Work out the finished part from the listing and answer in its coordinate system (mm). A direction names the side the tool comes from. Give positions to 0.01 mm unless a question says otherwise; leave off trailing zeros. Order: outer loops, then holes, each group sorted by start corner. A loop starts at its lowest first (then second) coordinate and runs counter-clockwise, first axis right, second up. Notation, with made-up numbers: (-30, 35.25) - (10, 35.25) arc R11 cw to (10, 49.25) - close; hole circle Ø8 at (77, -37.75). An arc over 180 degrees is marked (long way). Put each result on its own line as item: value.
```python
from build123d import *

# Parameters (mm, degrees)
SKETCH_1_R             = 1.6
SM_BASE_FLANGE_1_DEPTH = 0.9
OTHER_START            = -10
OTHER_1_DEPTH          = 20
OTHER_1_2_DEPTH        = 20


# Read off the part's stored shape, not the designer's step: 褶边1
# Sheet-metal steps are written as plain solids
with BuildPart() as part:
    # Sketch 1 → 基体-法兰1 (new body)
    with BuildSketch(Plane.XY):
        with BuildLine():
            Line((10, 0), (-10, 0))
            Line((-10, 0), (-10, 10))
            ThreePointArc((-10, 10), (0, 14.142135624), (10, 10))
            Line((10, 10), (10, 0))
        make_face()
        with Locations((-6.5, 6.5)):
            Circle(SKETCH_1_R, mode=Mode.SUBTRACT)
        with Locations(Location((6.5, 6.5, 0), (0, 0, 180))):
            Circle(SKETCH_1_R, mode=Mode.SUBTRACT)
    extrude(amount=-SM_BASE_FLANGE_1_DEPTH)

    # Other 1 outline → Other 1 (cut)
    with BuildSketch(Plane.YZ.offset(OTHER_START)):
        with BuildLine():
            ThreePointArc((2.4, -0.9), (1.360769515, -0.663330765), (0.5265006, 0))
            Line((0.5265006, 0), (0, 0))
            Line((0, 0), (0, -0.9))
            Line((0, -0.9), (2.4, -0.9))
        make_face()
    extrude(amount=OTHER_1_DEPTH, mode=Mode.SUBTRACT)

    # Other 1 2 outline → Other 1 2 (add)
    with BuildSketch(Plane.YZ.offset(OTHER_START)):
        with BuildLine():
            Line((2.4, 3), (2.4, 3.9))
            ThreePointArc((2.4, 3.9), (0.236669235, 2.539230485), (0.5265006, 0))
            Line((0.5265006, 0), (2.4, 0))
            ThreePointArc((2.4, 0), (0.9, 1.5), (2.4, 3))
        make_face()
    extrude(amount=OTHER_1_2_DEPTH)


solid = part.part
```
(1) Section A-A, the plane y = 6.5 is taken. Write down the section's boundary in (x, z), then the cut area to 3 significant figures.
Geometry check:
outline: (-10, -0.9) - (-8.1, -0.9) - (-8.1, 0) - (-10, 0) - close; (-4.9, -0.9) - (4.9, -0.9) - (4.9, 0) - (-4.9, 0) - close; (8.1, -0.9) - (10, -0.9) - (10, 0) - (8.1, 0) - close
area: 12.2 mm²
(2) A tool of negligible diameter and unlimited length cuts with its end or side. For faces 1 (the face through (-0.1, 2.4, 3.4)), 2 (the face through (5.76, 7.92, -0.44)), from which of +Z, -Z, +X, -X, +Y, -Y can it reach the whole face along a straight path? Write none if from no direction.
Geometry check:
face 1: +Z, +X, -X, +Y
face 2: +Z, -Z
(3) Straight lines are drawn through the part: line 1 (Z direction, x = 3.25, y = 9); line 2 (Y direction, x = 6.5, z = -0.25); line 3 (Y direction, x = 5.75, z = -0.6). For each, find the intervals that lie inside material, in ascending order.
Geometry check:
line 1: z = -0.9 to 0
line 2: y = 0.76 to 4.9, 8.1 to 12.56
line 3: y = 1.24 to 5.09, 7.91 to 12.92
(4) Section B-B, the plane x = -6.5 is taken. Write down the section's boundary in (y, z), then the cut area to 3 significant figures.
Geometry check:
outline: (2.4, -0.9) - (4.9, -0.9) - (4.9, 0) - (2.4, 0) arc R1.5 cw to (2.4, 3) - (2.4, 3.9) arc R2.4 ccw to start; (8.1, -0.9) - (12.56, -0.9) - (12.56, 0) - (8.1, 0) - close
area: 11.8 mm²
(5) Section D-D, the plane z = -0.5 is taken. Write down the section's boundary in (x, y), then the cut area to 3 significant figures.
Geometry check:
outline: (-10, 1.07) - (10, 1.07) - (10, 10) arc R14.14 ccw to (-10, 10) - close; hole circle Ø3.2 at (-6.5, 6.5); hole circle Ø3.2 at (6.5, 6.5)
area: 220 mm²
(6) Section C-C, the plane x = 1 is taken. Write down the section's boundary in (y, z).
Geometry check:
outline: (2.4, -0.9) - (14.11, -0.9) - (14.11, 0) - (2.4, 0) arc R1.5 cw to (2.4, 3) - (2.4, 3.9) arc R2.4 ccw to start
(7) Determine the mould class of faces 3 (the face through (-10, 4.2, -0.3)), 4 (the face through (-6.85, 4.94, -0.44)), 5 (the face through (-0.16, 14.14, -0.44)) for opening direction Y: pulls with the +Y half, pulls with the -Y half, needs draft (parallel to the pull), parting line crosses it, or undercut.
Geometry check:
face 3: needs draft
face 4: undercut
face 5: pulls with the +Y half
(8) Given pin 1 (6 mm diameter, centred on x = -1, y = 10, fed in from +Z), flat-ended and moving along its own axis, determine where the tip first touches the part or whether it passes through.
Geometry check:
pin 1: stops at z = 0
